Could you check a few things on this model? Use its own coordinates, in mm. A direction names the side the tool comes from. Round coordinates to 2 decimals unless told otherwise and drop trailing zeros. Order: outer loops, then holes, each group sorted by start corner. A loop starts at its lowest first (then second) coordinate and runs counter-clockwise, first axis right, second up. Notation, with made-up numbers: M 23.25,-10 L 32.25,-10 A26 ccw 32.25,9 Z; hole C -34.5,-12 d2. An arc over 180 degrees is marked long. Write each question's results on one line, items separated by ' | '. Start each with the question number.
1. Suppose I cut it at A-A on y = 0. Write out the boundary of the cut face in (x, z), and give its area (3 significant figures).
2. Please list where these lines run through material, in increasing order: L1, parallel to Y at x = 0, z = 6.4; L2, parallel to Z at x = 12, y = 4.5; L3, parallel to X at y = -10, z = -6.
3. Suppose I cut it at B-B on z = -5.75. Write out the boundary of the cut face in (x, y), and give its area (3 significant figures).
4. For faces 1 (the cylindrical face through (-22.496, 0.401, 0.105)), 2 (the cylindrical face through (1.216, 18.712, -1.115)), 3 (the cylindrical face through (10.17, -9.33, -0.06)), which set-ups out of +Z, -Z, +X, -X, +Y, -Y let a thin tool reach every point of the face, with its end or its side?
5. Suppose I cut it at C-C on y = -17.5. Write out the boundary of the cut face in (x, z), and give its area (3 significant figures).
6. We'd pull the mould along X, two halves only. Please class faces 4 (the cylindrical face through (22.496, -0.401, 0.105)), 5 (the flat face through (-10, 9, 7.5)), 6 (the cylindrical face through (-0.54, -18.71, 2.44)): released by +X, released by -X, zero draft, split by the parting line, or undercut.
7. Suppose I cut it at D-D on y = 9. Give the number of separate pieces and of enclosed holes in the cut face, and give its area (3 significant figures).
8. I'm going to push flat-ended pins straight in: pin 1 (4 mm diameter, centred on y = -4.5, z = 3.5, fed in from -X); pin 2 (2 mm diameter, centred on y = 7, z = -5.5, fed in from +X); pin 3 (1 mm diameter, centred on x = 0.5, z = -0.5, fed in from +Y); pin 4 (8.5 mm diameter, centred on x = 2.5, y = 5.5, fed in from -Z). Where does each tip first touch, or does it pass through?
from build123d import *

# Parameters (mm, degrees)
SKETCH_2_W                       = 64.02174429
SKETCH_2_H                       = 9.248919907
CUT_EXTRUDE_1_DEPTH              = 49
HOLE_WIZARD_M4_2_D               = 3.3
HOLE_WIZARD_M4_2_DEPTH           = 5.5
HOLE_WIZARD_M4_2_TIP             = 0.991420021
HOLE_WIZARD_M6_2_D               = 5
HOLE_WIZARD_M6_2_DEPTH           = 5.5
HOLE_WIZARD_M6_2_TIP             = 1.502151548
HOLE_WIZARD_M4_3_D               = 3.3
HOLE_WIZARD_M4_3_DEPTH           = 13.4
HOLE_WIZARD_M4_3_TIP             = 0.991420021
HOLE_WIZARD_M4_3_ON_FACE_2_D     = 3.3
HOLE_WIZARD_M4_3_ON_FACE_2_DEPTH = 13.4
HOLE_WIZARD_M4_3_ON_FACE_2_TIP   = 0.991420021


with BuildPart() as part:
    # 草图1 → 旋转1 (revolve)
    with BuildSketch(Plane(origin=(0, 0, 0), x_dir=(1, 0, 0), z_dir=(0, 1, 0)), mode=Mode.PRIVATE) as revolve_1_sk:
        Polygon((22.5, 7.5), (22.5, -7.5), (12.7, -7.5), (12.7, -4), (13.8, -4), (13.8, 4), (12.7, 4), (12.7, 7.5), align=None)
    revolve(revolve_1_sk.sketch.rotate(Axis((0, 0, -31.9390681), (0, 0, 1)), 180), axis=Axis((0, 0, -31.9390681), (0, 0, 1)))  # turned: the seam where the file's is

    # 草图2 → 切除-拉伸1 (cut)
    with BuildSketch(Plane.XY.offset(7.5)):
        with Locations((-1.141100508, 26.124459954)):
            Rectangle(SKETCH_2_W, SKETCH_2_H)
        with Locations((-1.141100508, -26.124459954)):
            Rectangle(SKETCH_2_W, SKETCH_2_H)
    extrude(amount=-CUT_EXTRUDE_1_DEPTH, mode=Mode.SUBTRACT)

    # M4 螺纹孔2
    with Locations(Plane(origin=(0, 21.5, 0), x_dir=(1, 0, 0), z_dir=(0, 1, 0))):
        with Locations((0, 0)):
            Hole(HOLE_WIZARD_M4_2_D / 2, depth=HOLE_WIZARD_M4_2_DEPTH)
            with Locations((0, 0, -(HOLE_WIZARD_M4_2_DEPTH + HOLE_WIZARD_M4_2_TIP / 2))):  # 118° drill point
                Cone(0, HOLE_WIZARD_M4_2_D / 2, HOLE_WIZARD_M4_2_TIP, mode=Mode.SUBTRACT)

    # M6 螺纹孔2
    with Locations(Plane(origin=(0, -21.5, 0), x_dir=(-1, 0, 0), z_dir=(0, -1, 0))):
        with Locations((0, 0)):
            Hole(HOLE_WIZARD_M6_2_D / 2, depth=HOLE_WIZARD_M6_2_DEPTH)
            with Locations((0, 0, -(HOLE_WIZARD_M6_2_DEPTH + HOLE_WIZARD_M6_2_TIP / 2))):  # 118° drill point
                Cone(0, HOLE_WIZARD_M6_2_D / 2, HOLE_WIZARD_M6_2_TIP, mode=Mode.SUBTRACT)

    # M4 螺纹孔3
    with Locations(Plane(origin=(19.485571585, 11.25, 0), x_dir=(-0.5, 0.866025404, 0), z_dir=(0.866025404, 0.5, 0))):
        with Locations((0, 0)):
            Hole(HOLE_WIZARD_M4_3_D / 2, depth=HOLE_WIZARD_M4_3_DEPTH)
            with Locations((0, 0, -(HOLE_WIZARD_M4_3_DEPTH + HOLE_WIZARD_M4_3_TIP / 2))):  # 118° drill point
                Cone(0, HOLE_WIZARD_M4_3_D / 2, HOLE_WIZARD_M4_3_TIP, mode=Mode.SUBTRACT)

    # M4 螺纹孔3 on face 2
    with Locations(Plane(origin=(-19.485571585, 11.25, 0), x_dir=(-0.500000175, -0.866025303, 0), z_dir=(-0.866025303, 0.500000175, 0))):
        with Locations((0, 0)):
            Hole(HOLE_WIZARD_M4_3_ON_FACE_2_D / 2, depth=HOLE_WIZARD_M4_3_ON_FACE_2_DEPTH)
            with Locations((0, 0, -(HOLE_WIZARD_M4_3_ON_FACE_2_DEPTH + HOLE_WIZARD_M4_3_ON_FACE_2_TIP / 2))):  # 118° drill point
                Cone(0, HOLE_WIZARD_M4_3_ON_FACE_2_D / 2, HOLE_WIZARD_M4_3_ON_FACE_2_TIP, mode=Mode.SUBTRACT)


solid = part.part
Filled sheet:
1) outline: M -22.5,-7.5 L -12.7,-7.5 L -12.7,-4 L -13.8,-4 L -13.8,4 L -12.7,4 L -12.7,7.5 L -22.5,7.5 Z; M 12.7,-7.5 L 22.5,-7.5 L 22.5,7.5 L 12.7,7.5 L 12.7,4 L 13.8,4 L 13.8,-4 L 12.7,-4 Z | area: 276 mm^2
2) L1: y = -21.5 to -12.7, 12.7 to 21.5 | L2: z = -7.5 to -4, 4 to 7.5 | L3: x = -20.16 to -7.83, 7.83 to 20.16
3) outline: M -6.63,-21.5 L 6.63,-21.5 A22.5 ccw 6.63,21.5 L -6.63,21.5 A22.5 ccw Z; hole C 0,0 d25.4 | area: 1,070 mm^2
4) face 1: +Z, -Z, -X | face 2: +Y | face 3: none
5) outline: M -14.14,-7.5 L 14.14,-7.5 L 14.14,7.5 L -14.14,7.5 Z; hole C 0,0 d5 | area: 405 mm^2
6) face 4: released by +X | face 5: zero draft | face 6: undercut
7) separate pieces: 2 | enclosed holes: 2 | area: 292 mm^2
8) pin 1: stops at x = -22.36 | pin 2: stops at x = 21.69 | pin 3: stops at y = 15.73 | pin 4: passes through
